Read the model definition and answer for the solid it produces. Units are mm, in the model's axes. A direction names the side the tool comes from. Coordinates: 2 decimals unless noted, no trailing zeros. Write each loop counter-clockwise with the first axis right and the second up, starting at its lowest first coordinate (ties: lowest second). Pieces come first, ordered by that corner, then holes. Notation, with made-up numbers: (1.25, 70) -> (25.25, 70) arc R19 cw to (25.25, 102) -> close; hole circle Ø6 at (31, 65). An arc over 180 degrees is marked (long way). Answer in a Markdown table with one row per item. Add a question column.
Item 1: Which of the six approach directions +Z, -Z, +X, -X, +Y, -Y give full straight-line access (tool end or side, diameter ignored) to faces 1 (the face through (-190, 75, -3)), 2 (the face through (-189.9, 70.5, 5.283)), 3 (the face through (-190, 66, 0))?
Item 2: Section D-D on y = 63 is taken. Write down the section's boundary in (x, z), then the cut area to 3 significant figures.
Item 3: Given pin 1 Ø1.6 at (x, y) = (-190.5, 66) entering from -Z; pin 2 Ø1.3 at (x, y) = (-189, 70) entering from +Z; pin 3 Ø1.3 at (x, y) = (-190, 70) entering from -Z; pin 4 Ø1.5 at (x, y) = (-191, 68.5) entering from -Z, each flat-ended and moving along its own axis, determine where each tip first touches the part or whether it passes through.
Item 4: Straight lines are drawn through the part: line 1 (Y direction, x = -191.5, z = 1); line 2 (Y direction, x = -191.6, z = 15); line 3 (Z direction, x = -190.4, y = 68.5). For each, find the intervals that lie inside material, in ascending order. Write a range as from..to.
Item 5: Section A-A on z = 3 is taken. Write down the section's boundary in (x, y).
Item 6: Section B-B on y = 67.5 is taken. Write down the section's boundary in (x, z), then the cut area to 3 significant figures.
Item 7: For a pull along Y with two mould halves and no side action, classify faces 4 (the face through (-189.9, 70.5, 3.483)), 5 (the face through (-190, 58.413, 6)), 6 (the face through (-190, 78.413, 6)) as +Y half, -Y half, draft (parallel to the pull), parting line (faces both ways), or undercut.
Autodesk Inventor part; units mm, degrees
ref_plane "YZ Plane" through (0, 0, 0) normal (1, 0, 0) x (0, 1, 0)
ref_plane "XZ Plane" through (0, 0, 0) normal (0, 1, 0) x (-1, 0, 0)
ref_plane "XY Plane" through (0, 0, 0) normal (0, 0, 1) x (1, 0, 0)
sketch "Эскиз1" plane through (0, 0, 0) normal (0, 0, 1) x (1, 0, 0)
  line L0 (-186.8805, 58.4127) -> (-192.8805, 58.4127)
  line L1 (-192.8805, 58.4127) -> (-192.8805, 78.4127)
  line L2 (-192.8805, 78.4127) -> (-186.8805, 78.4127)
  line L3 (-186.8805, 78.4127) -> (-186.8805, 58.4127)
  line L4 (-192.8805, 65.9127) -> (-192.8805, 70.9127)
  point P0 (0, 0)
  point P1 (-192.8805, 68.4127)
  dimension "d0" = 20
  dimension "d1" = 6
  dimension "d19" = 0
extrude "Выдавливание1" add sketch "Эскиз1" along normal blind 25
fillet "Сопряжение1" radius 10 2 edges at (-189.8805, 58.4127, 25) (-189.8805, 78.4127, 25)
sketch "Эскиз2" plane through (-192.8805, 58.4127, 0) normal (-1, 0, 0) x (0, 0, 1)
  circle A0 centre (15, 10) radius 1.9
  line L0 (0, 20) -> (0, 0)
  line L1 (0, 10) -> (25, 10) construction
  arc A1 (15, 0) -> (15, 20) centre (15, 10) ccw
  point P0 (0, -58.4127)
  dimension "d5" = 3.8
extrude "Выдавливание2" cut sketch "Эскиз2" against normal up to surface (6 mm away)
sketch "Эскиз3" plane through (0, 0, 0) normal (0, 0, -1) x (-1, 0, 0)
  line L0 (192.8805, 58.4127) -> (186.8805, 58.4127)
  line L1 (186.8805, 58.4127) -> (186.8805, 65.4127)
  line L2 (186.8805, 65.4127) -> (192.8805, 65.4127)
  line L3 (192.8805, 65.4127) -> (192.8805, 58.4127)
  line L4 (186.8805, 78.4127) -> (192.8805, 78.4127)
  line L5 (186.8805, 78.4127) -> (192.8805, 78.4127)
  line L6 (192.8805, 78.4127) -> (192.8805, 71.4127)
  line L7 (192.8805, 71.4127) -> (186.8805, 71.4127)
  line L8 (186.8805, 71.4127) -> (186.8805, 78.4127)
  point P0 (0, 0)
  dimension "d8" = 7
  dimension "d9" = 7
  dimension "d18" = 6
extrude "Выдавливание3" add sketch "Эскиз3" along normal blind 2
sketch "Эскиз4" plane through (-192.8805, 68.4127, 15) normal (-1, 0, 0) x (0, 0, 1)
  line L0 (-15, 3) -> (-15, -3)
  line L1 (-15, 0) -> (-4.7, 0)
  line L2 (-4.7, 0) -> (-4.7, -1.5)
  line L3 (-15, -1.5) -> (-15, 0)
  line L4 (-4.7, 0) -> (-4.7, 1.5)
  line L5 (-10.2565, 0) -> (-12.2169, 0)
  line L6 (-11.5169, -1.5) -> (-11.5169, -2.7)
  line L7 (-11.5169, -2.7) -> (-9.7169, -2.7)
  line L8 (-9.7169, -2.7) -> (-9.7169, -1.5)
  line L9 (-11.5169, 1.5) -> (-11.5169, 2.7)
  line L10 (-11.5169, 2.7) -> (-9.7169, 2.7)
  line L11 (-9.7169, 2.7) -> (-9.7169, 1.5)
  line L12 (-4.7, -1.5) -> (-9.7169, -1.5)
  line L13 (-11.5169, -1.5) -> (-15, -1.5)
  line L14 (-4.7, 1.5) -> (-9.7169, 1.5)
  line L15 (-11.5169, 1.5) -> (-15, 1.5)
  line L16 (-4.7, 1.5) -> (-9.7169, 1.5)
  line L17 (-11.5169, 1.5) -> (-15, 1.5)
  point P0 (-15, -68.4127)
  dimension "d12" = 10.3
  dimension "d13" = 1.5
  dimension "d16" = 1.8
  dimension "d17" = 5.4
extrude "Выдавливание4" cut sketch "Эскиз4" against normal up to surface (6 mm away)
sketch "Эскиз5" plane through (0, 0, -2) normal (0, 0, -1) x (-1, 0, 0)
  point P0 (0, 0)
sketch "Эскиз6" plane through (0, 0, -2) normal (0, 0, -1) x (-1, 0, 0)
  line L0 (186.8805, 71.4127) -> (192.8805, 71.4127)
  line L1 (192.8805, 71.4127) -> (192.8805, 78.4127)
  line L2 (192.8805, 78.4127) -> (186.8805, 78.4127)
  line L3 (186.8805, 78.4127) -> (186.8805, 71.4127)
  line L4 (192.8805, 65.4127) -> (186.8805, 65.4127)
  line L5 (186.8805, 65.4127) -> (186.8805, 58.4127)
  line L6 (186.8805, 58.4127) -> (192.8805, 58.4127)
  line L7 (192.8805, 58.4127) -> (192.8805, 65.4127)
  point P0 (0, 0)
sketch "Эскиз7" plane through (0, 0, -2) normal (0, 0, -1) x (-1, 0, 0)
  point P0 (0, 0)
extrude "Выдавливание5" add sketch "Эскиз6" along normal blind 1
properties part number "Крепление рычага к лицу"
Results below:
| question | item | result |
|---|---|---|
| 1 | face 1 | -Z, +X, -X, +Y, -Y |
| 1 | face 2 | +X, -X |
| 1 | face 3 | -Z, +X, -X |
| 2 | outline | (-192.88, -3) -> (-186.88, -3) -> (-186.88, 23.41) -> (-192.88, 23.41) -> close |
| 2 | area | 158 mm2 |
| 3 | pin 1 | stops at z = -3 |
| 3 | pin 2 | stops at z = 24.96 |
| 3 | pin 3 | stops at z = 0 |
| 3 | pin 4 | stops at z = 10.3 |
| 4 | line 1 | y = 58.41..66.91, 69.91..78.41 |
| 4 | line 2 | y = 58.41..66.51, 70.31..78.41 |
| 4 | line 3 | z = 10.3..13.1, 16.9..25 |
| 5 | outline | (-192.88, 58.41) -> (-186.88, 58.41) -> (-186.88, 66.91) -> (-192.88, 66.91) -> close; (-192.88, 69.91) -> (-186.88, 69.91) -> (-186.88, 78.41) -> (-192.88, 78.41) -> close |
| 6 | outline | (-192.88, 10.3) -> (-186.88, 10.3) -> (-186.88, 13.33) -> (-192.88, 13.33) -> close; (-192.88, 16.67) -> (-186.88, 16.67) -> (-186.88, 24.96) -> (-192.88, 24.96) -> close |
| 6 | area | 68.0 mm2 |
| 7 | face 4 | undercut |
| 7 | face 5 | -Y half |
| 7 | face 6 | +Y half |
